Input: part model. Units: mm. Frame: model coordinates. Give positions to 0.01 mm unless a question says otherwise; leave off trailing zeros. Loops run counter-clockwise (first coordinate to the right, second up) from the corner with the lowest first, then second, coordinate; pieces in that order, holes last. Notation, with made-up numbers: M 9.25,-1 L 63.25,-1 A15 cw 63.25,11 Z; hole C -35.5,67 d8. An arc over 180 degrees is marked long. Use a Markdown table: item, result. Add a question column.
from build123d import *

# Parameters (mm, degrees)
SKETCH2_W           = 200
SKETCH2_H           = 130
BOSS_EXTRUDE1_DEPTH = 3.18
SKETCH5_W           = 7
SKETCH5_H           = 3.18
BOSS_EXTRUDE2_DEPTH = 3.18
SKETCH11_R          = 1.47
CUT_EXTRUDE5_DEPTH  = 3.18


with BuildPart() as part:
    # Sketch2 → Boss-Extrude1 (new body)
    with BuildSketch(Plane(origin=(0, 0, 0), x_dir=(1, 0, 0), z_dir=(0, 1, 0))):
        Rectangle(SKETCH2_W, SKETCH2_H)
    extrude(amount=BOSS_EXTRUDE1_DEPTH)

    # Sketch5 → Boss-Extrude2 (add)
    with BuildSketch(Plane.ZY.offset(100)):
        with Locations((0, 1.59)):
            Rectangle(SKETCH5_W, SKETCH5_H)
    boss_extrude2 = extrude(amount=BOSS_EXTRUDE2_DEPTH)

    # Sketch11 → Cut-Extrude5 (cut)
    with BuildSketch(Plane(origin=(0, 3.18, 0), x_dir=(1, 0, 0), z_dir=(0, 1, 0))):
        with Locations((-101.55, 0)):
            Circle(SKETCH11_R)
    cut_extrude5 = extrude(amount=-CUT_EXTRUDE5_DEPTH, mode=Mode.SUBTRACT)

    # Mirror1: Boss-Extrude2, Cut-Extrude5 across plane
    add(boss_extrude2.mirror(Plane(origin=(0, 0, 0), x_dir=(0, 0, 1), z_dir=(1, 0, 0))))
    add(cut_extrude5.mirror(Plane(origin=(0, 0, 0), x_dir=(0, 0, 1), z_dir=(1, 0, 0))), mode=Mode.SUBTRACT)


solid = part.part
1) Section query B-B, the plane z = -6. Return the cut outline in (x, y), and give its area (3 significant figures).
2) Section query A-A, the plane y = 2.45. Return the cut outline in (x, z), and give its area (3 significant figures).
3) Ray query, line 1 (X direction, y = 1.5, z = 0); line 2 (Z direction, x = -101.55, y = 2.3); line 3 (X direction, y = 1.25, z = -1). Return the intervals inside material, ascending. Write a range as [from, to].
4) Contact query for flat-ended pins moving along their axis: P1, Ø1.6, axis at x = -101.5, y = 2, coming from the -Z side; P2, Ø2.5, axis at x = -101.55, z = 0, coming from the +Y side; P3, Ø1.6, axis at y = 1.5, z = 37.5, coming from the +X side; P4, Ø1.6, axis at y = 1, z = 35, coming from the -X side. Output: stop coordinate, or through.
Entries:
| question | item | result |
|---|---|---|
| 1 | outline | M -100,0 L 100,0 L 100,3.18 L -100,3.18 Z |
| 1 | area | 636 mm² |
| 2 | outline | M -103.18,-3.5 L -100,-3.5 L -100,-65 L 100,-65 L 100,-3.5 L 103.18,-3.5 L 103.18,3.5 L 100,3.5 L 100,65 L -100,65 L -100,3.5 L -103.18,3.5 Z; hole C -101.55,0 d2.94; hole C 101.55,0 d2.94 |
| 2 | area | 26,000 mm² |
| 3 | line 1 | x = [-103.18, -103.02], [-100.08, 100.08], [103.02, 103.18] |
| 3 | line 2 | z = [-3.5, -1.47], [1.47, 3.5] |
| 3 | line 3 | x = [-103.18, -102.63], [-100.47, 100.47], [102.63, 103.18] |
| 4 | P1 | stops at z = -3.5 |
| 4 | P2 | passes through |
| 4 | P3 | stops at x = 100 |
| 4 | P4 | stops at x = -100 |
